Autodesk Inventor part; units mm, degrees
ref_plane "YZ Plane" through (0, 0, 0) normal (1, 0, 0) x (0, 1, 0)
ref_plane "XZ Plane" through (0, 0, 0) normal (0, 1, 0) x (-1, 0, 0)
ref_plane "XY Plane" through (0, 0, 0) normal (0, 0, 1) x (1, 0, 0)
sketch "草图1" plane through (0, 0, 0) normal (0, 1, 0) x (-1, 0, 0)
  circle A0 centre (0, 0) radius 11
  circle A1 centre (0, 0) radius 3.5
  circle A2 centre (0, 0) radius 7
  circle A3 centre (7, 0) radius 1.525
  circle A4 centre (0, 7) radius 1.525
  circle A5 centre (-7, 0) radius 1.525
  circle A6 centre (0, -7) radius 1.525
  line L0 (0, 0) -> (2.6058, 0)
  line L1 (0, 0) -> (0, -1.55)
  line L2 (-0.8049, 10.9705) -> (-41.5854, 7.9786)
  line L3 (-41.5854, 7.9786) -> (-41.5854, -7.9786)
  line L4 (-41.5854, -7.9786) -> (-0.8049, -10.9705)
  circle A7 centre (-41, 0) radius 8
  circle A8 centre (-41, 0) radius 4.15
  point P0 (-41.5854, -7.9786)
  dimension "d7" = 16
  dimension "d0" = 22
  dimension "d1" = 7
  dimension "d2" = 14
  dimension "d3" = 3.05
  dimension "d4" = 3.05
  dimension "d5" = 3.05
  dimension "d6" = 3.05
  dimension "d8" = 41
  dimension "d9" = 8.3
extrude "拉伸1" add sketch "草图1" along normal blind 5 contours A0 | A0 L4 A7 L2 | A7 L3 A8 | L3 A8 A7 | A3 A2 A6 A5 A4
properties part number "leg4"
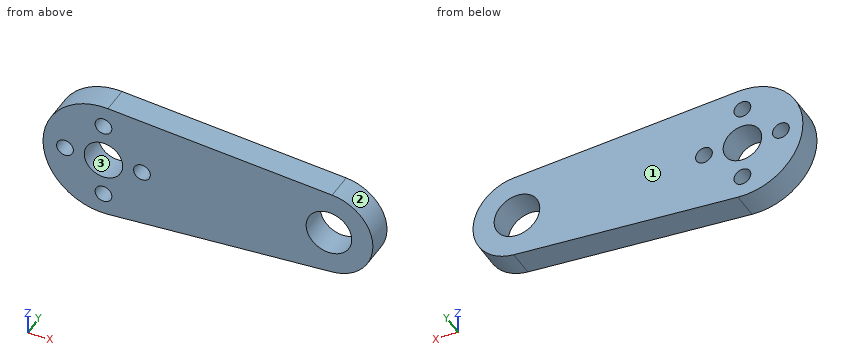
Read the model definition and answer for the solid it produces. Units are mm, in the model's axes. Face numbers are marked on the shaded views. Give positions to 0.01 mm unless a question says otherwise; leave off trailing zeros. Write each loop counter-clockwise with the first axis right and the second up, starting at its lowest first coordinate (ties: lowest second). Pieces come first, ordered by that corner, then holes. Notation, with made-up numbers: (35, 85) - (74, 85) arc R16 cw to (74, 97) - close; hole circle Ø3 at (-6.5, 76.5). An arc over 180 degrees is marked (long way). Use CSV: the item, a comma, the result in double quotes. Start each with the question number.
Item 1: The part is cut by section C-C, the plane y = 0.65. Count the separate pieces of the cut face and the enclosed holes in it, and give its area (3 significant figures).
Item 2: Flat-ended cylindrical pins translate along their axes: P1, Ø2, axis at x = 19.5, y = 3.5, coming from the -Z side; P2, Ø2, axis at y = 3.5, z = 1.5, coming from the +X side; P3, Ø3, axis at y = 4, z = 7.5, coming from the -X side. Find the tip coordinate at first contact, or state that the pin passes through.
Item 3: Consider line 1 (Z direction, x = 0, y = 3.65) (3 decimals); line 2 (Z direction, x = 1, y = 4.7); line 3 (X direction, y = 3.4, z = 3). Determine where each line is inside the solid, lowest interval first.
Item 4: The part is cut by section A-A, the plane x = 0. Give the vertices of the cut face in (y, z) (3 decimals), and give its area (3 significant figures).
Item 5: The part is cut by section D-D, the plane x = 40. Give the vertices of the cut face in (y, z), and give its area (3 significant figures).
Item 6: The part is cut by section B-B, the plane z = -7. Give the vertices of the cut face in (x, y) (3 decimals), and give its area (3 significant figures).
Item 7: The mould has two halves that part along Z. Classify the marked faces 1, 2 and 3: pulls with the +Z half, pulls with the -Z half, needs draft (parallel to the pull), parting line crosses it, or undercut.
Taken from the geometry:
1,separate pieces,"1"
1,enclosed holes,"6"
1,area,"950 mm2"
2,P1,"z = -9.67"
2,P2,"x = 48.98"
2,P3,"x = -9.22"
3,line 1,"-11 to -8.525, -5.475 to -3.5, 3.5 to 5.475, 8.525 to 11"
3,line 2,"-10.96 to -8.15, -5.85 to -3.35, 3.35 to 5.85, 8.15 to 10.96"
3,line 3,"-10.58 to -1.8, 1.8 to 38.13, 43.87 to 48.42"
4,outline,"(0, -11) - (5, -11) - (5, -8.525) - (0, -8.525) - close; (0, -5.475) - (5, -5.475) - (5, -3.5) - (0, -3.5) - close; (0, 3.5) - (5, 3.5) - (5, 5.475) - (0, 5.475) - close; (0, 8.525) - (5, 8.525) - (5, 11) - (0, 11) - close"
4,area,"44.5 mm2"
5,outline,"(0, -8.09) - (5, -8.09) - (5, -4.03) - (0, -4.03) - close; (0, 4.03) - (5, 4.03) - (5, 8.09) - (0, 8.09) - close"
5,area,"40.7 mm2"
6,outline,"(-8.485, 0) - (-1.525, 0) - (-1.525, 5) - (-8.485, 5) - close; (1.525, 0) - (44.873, 0) - (44.873, 5) - (1.525, 5) - close"
6,area,"252 mm2"
7,face 1,"needs draft"
7,face 2,"parting line crosses it"
7,face 3,"undercut"
